Input: part model. Units: mm. Frame: model coordinates. A direction names the side the tool comes from. Give positions to 0.01 mm unless a question says otherwise; leave off trailing zeros. Loops run counter-clockwise (first coordinate to the right, second up) from the corner with the lowest first, then second, coordinate; pieces in that order, holes last. Notation, with made-up numbers: (71.25, 5.5) - (127.25, 5.5) arc R17 ccw to (127.25, 16.5) - close; hole circle Ø2 at (27, 81.5). An arc over 180 degrees is marked (long way). Answer as a JSON object with one key per item and string values.
from build123d import *

# Parameters (mm, degrees)
F1_DEPTH = 19.05
F2_R     = 1.5875
F3_DEPTH = 1.651


with BuildPart() as f1:
    # F0 (on Front) → F1 (new body)
    with BuildSketch(Plane.XZ):
        with BuildLine():
            Line((0, 3.175), (0, 0))
            ThreePointArc((0, 0), (-0.36356, -0.690866), (-1.138859, -0.782422))
            Line((-1.138859, -0.782422), (-3.175, 0))
            Line((-3.175, 0), (-11.811, 0))
            ThreePointArc((-11.811, 0), (-12.439618, -0.260382), (-12.7, -0.889))
            Line((-12.7, -0.889), (-12.7, -2.286))
            ThreePointArc((-12.7, -2.286), (-12.439618, -2.914618), (-11.811, -3.175))
            Line((-11.811, -3.175), (-0.8382, -3.175))
            ThreePointArc((-0.8382, -3.175), (1.406864, -2.245064), (2.3368, 0))
            Line((2.3368, 0), (2.3368, 3.175))
            ThreePointArc((2.3368, 3.175), (1.406864, 5.420064), (-0.8382, 6.35))
            Line((-0.8382, 6.35), (-11.811, 6.35))
            ThreePointArc((-11.811, 6.35), (-12.439618, 6.089618), (-12.7, 5.461))
            Line((-12.7, 5.461), (-12.7, 4.064))
            ThreePointArc((-12.7, 4.064), (-12.439618, 3.435382), (-11.811, 3.175))
            Line((-11.811, 3.175), (-3.175, 3.175))
            Line((-3.175, 3.175), (-1.138859, 3.957422))
            ThreePointArc((-1.138859, 3.957422), (-0.36356, 3.865866), (0, 3.175))
        make_face()
    extrude(amount=F1_DEPTH)

    # F2 (on face) → F3 (cut)
    with BuildSketch(Plane(origin=(0, 0, -3.175), x_dir=(1, 0, 0), z_dir=(0, 0, -1))):
        with Locations((-6.35, 15.875)):
            Circle(F2_R)
        with Locations((-6.35, 3.175)):
            Circle(F2_R)
        with Locations((-6.35, 9.525)):
            Circle(F2_R)
    extrude(amount=-F3_DEPTH, mode=Mode.SUBTRACT)


solid = f1.part
Item 1: Cut plane D-D (x = -9.25). Return loops of the section in (y, z) (3 decimals), then the cut area to 3 significant figures.
Geometry check:
{"outline": "(-19.05, -3.175) - (0, -3.175) - (0, 0) - (-19.05, 0) - close; (-19.05, 3.175) - (0, 3.175) - (0, 6.35) - (-19.05, 6.35) - close", "area": "121 mm2"}
Item 2: Contact query for flat-ended pins moving along their axis: P1, Ø1.6, axis at x = -6.5, y = -9.5, coming from the -Z side; P2, Ø1, axis at x = 0, y = -12, coming from the -Z side; P3, Ø3, axis at y = -16.5, z = 3.5, coming from the -X side; P4, Ø1, axis at y = -8.5, z = 0, coming from the -X side. Output: stop coordinate, or through.
Geometry check:
{"P1": "stops at z = -1.52", "P2": "stops at z = -3.16", "P3": "stops at x = -12.7", "P4": "stops at x = -12.61"}
Item 3: Cut plane C-C (z = -0.25). Return loops of the section in (x, y).
Geometry check:
{"outline": "(-12.43, -19.05) - (-2.52, -19.05) - (-2.52, 0) - (-12.43, 0) - close; (-0.04, -19.05) - (2.33, -19.05) - (2.33, 0) - (-0.04, 0) - close"}
Item 4: Cut plane B-B (y = -17.75). Return loops of the section in (x, z) (3 decimals), then the cut area to 3 significant figures.
Geometry check:
{"outline": "(-12.7, -2.286) arc R0.889 ccw to (-11.811, -3.175) - (-0.838, -3.175) arc R3.175 ccw to (2.337, 0) - (2.337, 3.175) arc R3.175 ccw to (-0.838, 6.35) - (-11.811, 6.35) arc R0.889 ccw to (-12.7, 5.461) - (-12.7, 4.064) arc R0.889 ccw to (-11.811, 3.175) - (-3.175, 3.175) - (-1.139, 3.957) arc R0.838 cw to (0, 3.175) - (0, 0) arc R0.838 cw to (-1.139, -0.782) - (-3.175, 0) - (-11.811, 0) arc R0.889 ccw to (-12.7, -0.889) - close", "area": "94.7 mm2"}
Item 5: Access query for faces 5 (the face through (-12.43, -9.39, -0.25)), 6 (the face through (-6, -3, -1.524)), 7 (the face through (-0.37, -9.39, 3.87)), 8 (the face through (-12.7, -9, 5)), 9 (the face through (-6, -12, -3.175)). Directions: +Z, -Z, +X, -X, +Y, -Y. A direction counts if a zero-diameter tool reaches every point of the face in a straight line with its end or side. Return the directions, or none.
Geometry check:
{"face 5": "-X, +Y, -Y", "face 6": "-Z", "face 7": "+Y, -Y", "face 8": "+Z, -Z, -X, +Y, -Y", "face 9": "-Z, +X, -X, +Y, -Y"}
Item 6: Material intervals for line 1 (Y direction, x = -6.35, z = -1.95); line 2 (Z direction, x = -0.75, y = -3); line 3 (Z direction, x = -9.25, y = -6.25) (3 decimals), sorted ascending. Write a range as [from, to].
Geometry check:
{"line 1": "y = [-19.05, -17.46], [-14.29, -11.11], [-7.94, -4.76], [-1.59, 0]", "line 2": "z = [-3.17, -0.83], [4.01, 6.35]", "line 3": "z = [-3.175, 0], [3.175, 6.35]"}
Item 7: Mould query, pull axis X, two halves, no side actions, for faces 1 (the face through (-5, -19.05, 4)), 2 (the face through (-6, -16, -1.524)), 3 (the face through (-12.7, -9, -2)), 4 (the face through (-2.143, -9.392, -0.397)). Classes: released by +X, released by -X, zero draft, split by the parting line, or undercut.
Geometry check:
{"face 1": "zero draft", "face 2": "undercut", "face 3": "released by -X", "face 4": "undercut"}
